Design review of the part built by this model. Coordinates are the model's own, in mm. Give positions to 0.01 mm unless a question says otherwise; leave off trailing zeros. Write each loop counter-clockwise with the first axis right and the second up, starting at its lowest first coordinate (ties: lowest second). Pieces come first, ordered by that corner, then holes. Notation, with made-up numbers: (83.5, 65) -> (121.5, 65) arc R20 cw to (121.5, 102) -> close; hole circle Ø2 at (-36, 63). An arc over 180 degrees is marked (long way). Use CSV: the item, a comma, the result in double quotes.
Autodesk Inventor part; units mm, degrees
ref_plane "YZ Plane" through (0, 0, 0) normal (1, 0, 0) x (0, 1, 0)
ref_plane "XZ Plane" through (0, 0, 0) normal (0, 1, 0) x (-1, 0, 0)
ref_plane "XY Plane" through (0, 0, 0) normal (0, 0, 1) x (1, 0, 0)
sketch "Sketch1" plane through (0, 0, 0) normal (0, 1, 0) x (-1, 0, 0)
  line L0 (-8.255, 7.149) -> (8.255, 7.149) construction
  line L1 (8.255, 7.149) -> (0, -7.149) construction
  line L2 (0, -7.149) -> (-8.255, 7.149) construction
  line L3 (0, -7.149) -> (0, 7.149) construction
  circle A0 centre (-8.255, 7.149) radius 1.524 construction
  circle A1 centre (8.255, 7.149) radius 1.524 construction
  circle A2 centre (0, -7.149) radius 1.524 construction
  circle A3 centre (-8.255, 7.149) radius 0.381
  circle A4 centre (8.255, 7.149) radius 0.381
  circle A5 centre (0, -7.149) radius 0.381
  line L4 (-8.255, 10.324) -> (8.255, 10.324)
  line L5 (-11.0046, 5.5615) -> (-2.7496, -8.7365)
  line L6 (11.0046, 5.5615) -> (2.7496, -8.7365)
  arc A6 (-8.255, 10.324) -> (-11.0046, 5.5615) centre (-8.255, 7.149) ccw
  arc A7 (11.0046, 5.5615) -> (8.255, 10.324) centre (8.255, 7.149) ccw
  arc A8 (-2.7496, -8.7365) -> (2.7496, -8.7365) centre (0, -7.149) ccw
  line L7 (8.255, 7.149) -> (-4.1275, 0) construction
  line L8 (-8.255, 7.149) -> (4.1275, 0) construction
  circle A9 centre (0, 2.383) radius 0.381
  point P0 (0, 0)
  point P1 (0, 0)
  dimension "d1" = 16.51
  dimension "d2" = 3.048
  dimension "d3" = 0.762
  dimension "d4" = 3.175
  dimension "d5" = 0.762
extrude "Extrusion1" add sketch "Sketch1" along normal blind 6.35
properties part number "RollerMounter"
(1) Clearance check with flat-ended pins moving along their axes: pin 1 (1.5 mm diameter, centred on y = 4.5, z = 1, fed in from -X); pin 2 (3 mm diameter, centred on y = 3, z = -4.5, fed in from +X). State where each tip first meets the part, or that it passes through.
Established:
pin 1,"stops at x = -8.8"
pin 2,"stops at x = 6.06"
(2) For line 1 along X through (y, z) = (3, 7.25); line 2 along Z through (x, y) = (8, 4); line 3 along Z through (x, y) = (8.25, 6), list the stretches that pass through material, from the lowest coordinate up. Write a range as [from, to].
Established:
line 1,"x = [-11.43, -8.62], [-7.89, 7.89], [8.62, 11.43]"
line 2,"z = [0.36, 6.87], [7.43, 10.32]"
line 3,"z = [0.79, 6.77], [7.53, 10.32]"
(3) Take a section at B-B (y = 5). State how many separate pieces and enclosed holes the cut face has, then the cut area to 3 significant figures.
Established:
separate pieces,"1"
enclosed holes,"4"
area,"305 mm2"
(4) Take a section at D-D (x = 3.5). Write out the cut boundary in (y, z).
Established:
outline,"(0, -7.44) -> (6.35, -7.44) -> (6.35, 10.32) -> (0, 10.32) -> close"
(5) Take a section at A-A (x = 0). Write out the cut boundary in (y, z).
Established:
outline,"(0, -10.32) -> (6.35, -10.32) -> (6.35, -7.53) -> (0, -7.53) -> close; (0, -6.77) -> (6.35, -6.77) -> (6.35, 2) -> (0, 2) -> close; (0, 2.76) -> (6.35, 2.76) -> (6.35, 10.32) -> (0, 10.32) -> close"
(6) Mouldability with a two-part tool opening along X and no side actions: class faces 1 (the face through (-10.98, 3.13, 8.78)), 2 (the face through (0, 0, 5)), 3 (the face through (11.028, 3.131, 8.696)) as +X half, -X half, draft (parallel to the pull), parting line (faces both ways), or undercut.
Established:
face 1,"-X half"
face 2,"draft"
face 3,"+X half"
(7) Take a section at C-C (z = -3). Write out the cut boundary in (x, y), then the cut area to 3 significant figures.
Established:
outline,"(-6.06, 0) -> (6.06, 0) -> (6.06, 6.35) -> (-6.06, 6.35) -> close"
area,"77.0 mm2"
